from build123d import *

# Parameters (mm, degrees)
BOSS_EXTRUDE1_DEPTH = 96.03
SKETCH2_W           = 5.1054
SKETCH2_H           = 5.89375
SKETCH3_R           = 1.5
CUT_EXTRUDE1_DEPTH  = 98.178397291


with BuildPart() as part:
    # Sketch1 → Boss-Extrude1 (new, symmetric)
    with BuildSketch(Plane(origin=(0, 0, 0), x_dir=(0, 0, -1), z_dir=(1, 0, 0))):
        Polygon((7.447818473, 0), (3.723909236, 6.45), (-3.723909236, 6.45), (-7.447818473, 0), (-3.723909236, -6.45), (3.723909236, -6.45), align=None)
    extrude(amount=BOSS_EXTRUDE1_DEPTH, both=True)

    # Sketch2 → Cut-Revolve1 (revolve, cut)
    with BuildSketch(Plane.XY, mode=Mode.PRIVATE) as cut_revolve1_sk:
        with Locations((-88.4773, 8.503125)):
            Rectangle(SKETCH2_W, SKETCH2_H)
        with Locations((66.6281, 8.503125)):
            Rectangle(SKETCH2_W, SKETCH2_H)
    revolve(cut_revolve1_sk.sketch.rotate(Axis((-251.263286978, 0, 0), (1, 0, 0)), 90), axis=Axis((-251.263286978, 0, 0), (1, 0, 0)), mode=Mode.SUBTRACT)

    # Sketch3 → Cut-Extrude1 (cut, through all)
    with BuildSketch(Plane(origin=(0, 6.45, 0), x_dir=(1, 0, 0), z_dir=(0, 1, 0))):
        with Locations(Location((74.1808, 0, 0), (0, 0, 270))):
            Circle(SKETCH3_R)
        with Locations(Location((87.5308, 0, 0), (0, 0, 270))):
            Circle(SKETCH3_R)
    extrude(amount=-CUT_EXTRUDE1_DEPTH, mode=Mode.SUBTRACT)


solid = part.part
Design review of the part built by this model. Coordinates are the model's own, in mm. Give positions to 0.01 mm unless a question says otherwise; leave off trailing zeros. Loops run counter-clockwise (first coordinate to the right, second up) from the corner with the lowest first, then second, coordinate; pieces in that order, holes last. Notation, with made-up numbers: M 21.5,79.5 L 29.5,79.5 A23 ccw 29.5,112.5 Z; hole C 50.25,22.5 d11. An arc over 180 degrees is marked long. One line per question, with ' | ' between items. Start each with the question number.
1. Add section C-C (y = 3.75). Write out the cut boundary in (x, z), plus the area to 3 significant figures.
2. Add section B-B (x = -54.5). Write out the cut boundary in (y, z).
3. The part is to be moulded in two halves that separate along X. For faces 1 (the face through (83, 6.45, 0)), 2 (the face through (-96.03, 0, 0)), 3 (the face through (64.075, -3, -5)), say which applies: released by +X, released by -X, zero draft, split by the parting line, or undercut.
4. Insertion check: P1, Ø1, axis at x = -22, y = -4, coming from the -Z side; P2, Ø1.5, axis at x = -22, y = -2, coming from the -Z side; P3, Ø1, axis at x = 43.5, z = 4.5, coming from the +Y side. Each pin has a flat end and moves straight along its axis. Give the tip position at first contact, or say it passes through.
5. To check wall thickness, follow L1, parallel to X at y = -5, z = -2.5; L2, parallel to X at y = 1.5, z = 0; L3, parallel to Z at x = 82.5, y = -1.75. State the ranges of each line that lie inside material, in increasing order.
6. Add section A-A (y = -3.5). Write out the cut boundary in (x, z), plus the area to 3 significant figures.
Worked out:
1) outline: M -96.03,-5.28 L -91.03,-5.28 L -91.03,-4.1 L -85.92,-4.1 L -85.92,-5.28 L 64.08,-5.28 L 64.08,-4.1 L 69.18,-4.1 L 69.18,-5.28 L 96.03,-5.28 L 96.03,5.28 L 69.18,5.28 L 69.18,4.1 L 64.08,4.1 L 64.08,5.28 L -85.92,5.28 L -85.92,4.1 L -91.03,4.1 L -91.03,5.28 L -96.03,5.28 Z; hole C 74.18,0 d3; hole C 87.53,0 d3 | area: 1,990 mm²
2) outline: M -6.45,-3.72 L 0,-7.45 L 6.45,-3.72 L 6.45,3.72 L 0,7.45 L -6.45,3.72 Z
3) face 1: zero draft | face 2: released by -X | face 3: undercut
4) P1: stops at z = -5.43 | P2: stops at z = -6.73 | P3: stops at y = 5.97
5) L1: x = -96.03 to -91.03, -85.92 to 64.08, 69.18 to 96.03 | L2: x = -96.03 to 72.68, 75.68 to 86.03, 89.03 to 96.03 | L3: z = -6.44 to 6.44
6) outline: M -96.03,-5.43 L -91.03,-5.43 L -91.03,-4.32 L -85.92,-4.32 L -85.92,-5.43 L 64.08,-5.43 L 64.08,-4.32 L 69.18,-4.32 L 69.18,-5.43 L 96.03,-5.43 L 96.03,5.43 L 69.18,5.43 L 69.18,4.32 L 64.08,4.32 L 64.08,5.43 L -85.92,5.43 L -85.92,4.32 L -91.03,4.32 L -91.03,5.43 L -96.03,5.43 Z; hole C 74.18,0 d3; hole C 87.53,0 d3 | area: 2,050 mm²
